Verification items for the finished model (mm, model axes). Face numbers are marked on the shaded views. Coordinates: 2 decimals unless noted, no trailing zeros. Order: outer loops, then holes, each group sorted by start corner. A loop starts at its lowest first (then second) coordinate and runs counter-clockwise, first axis right, second up. Notation, with made-up numbers: M 28,-22.5 L 72,-22.5 A32 cw 72,7.5 Z; hole C 17,11 d7. An arc over 180 degrees is marked long. Return JSON: item names as keys, results as strings.
```python
from build123d import *

# Parameters (mm, degrees)
BOX002_W          = 3
BOX002_H          = 176
BOX002_DEPTH      = 26
FILLET001_R       = 2
CYLINDER020_R     = 30
CYLINDER020_DEPTH = 10
CYLINDER019_R     = 30
CYLINDER019_DEPTH = 10
CYLINDER018_R     = 30
CYLINDER018_DEPTH = 10
CYLINDER016_R     = 30
CYLINDER016_DEPTH = 10
CYLINDER017_R     = 70
CYLINDER017_DEPTH = 10
CYLINDER015_R     = 70
CYLINDER015_DEPTH = 10
CYLINDER014_R     = 70
CYLINDER014_DEPTH = 10
CYLINDER013_R     = 70
CYLINDER013_DEPTH = 10
BOX004_W          = 10
BOX004_H          = 24
BOX004_DEPTH      = 15
CYLINDER012_R     = 30
CYLINDER012_DEPTH = 10
CYLINDER011_R     = 30
CYLINDER011_DEPTH = 10
CYLINDER010_R     = 30
CYLINDER010_DEPTH = 10
CYLINDER008_R     = 30
CYLINDER008_DEPTH = 10
CYLINDER009_R     = 70
CYLINDER009_DEPTH = 10
CYLINDER006_R     = 70
CYLINDER006_DEPTH = 10
CYLINDER005_R     = 70
CYLINDER005_DEPTH = 10
CYLINDER004_R     = 70
CYLINDER004_DEPTH = 10
BOX003_W          = 10
BOX003_H          = 24
BOX003_DEPTH      = 15
BOX_W             = 2
BOX_H             = 176
BOX_DEPTH         = 26
CYLINDER_R        = 2
CYLINDER_DEPTH    = 26
CYLINDER001_R     = 2
CYLINDER001_DEPTH = 26
CYLINDER002_R     = 2
CYLINDER002_DEPTH = 176
CYLINDER003_R     = 2
CYLINDER003_DEPTH = 176
BOX001_W          = 3
BOX001_H          = 180
BOX001_DEPTH      = 30
FILLET_R          = 2


with BuildPart() as fillet001:
    # Box002 → Box002 (new body)
    with BuildSketch(Plane(origin=(7, 2, 2), x_dir=(1, 0, 0), z_dir=(0, 0, 1))):
        with Locations((1.5, 88)):
            Rectangle(BOX002_W, BOX002_H)
    extrude(amount=BOX002_DEPTH)

    # Fillet001
    fillet001_edges = [fillet001.edges().sort_by_distance(p)[0] for p in [
        (8.5, 2, 2),
        (8.5, 2, 28),
        (8.5, 178, 2),
        (8.5, 178, 28),
    ]]
    fillet(fillet001_edges, radius=FILLET001_R)


with BuildPart() as fillet001_1:
    # Fillet001 placement: moved
    add(fillet001.part.moved(Location((-5, 0, 0))))


with BuildPart() as cylinder020:
    # Cylinder020 → Cylinder020 (new body)
    with BuildSketch(Plane(origin=(22, -27, 39.5), x_dir=(0, 0, -1), z_dir=(1, 0, 0))):
        Circle(CYLINDER020_R)
    extrude(amount=CYLINDER020_DEPTH)


with BuildPart() as cylinder019:
    # Cylinder019 → Cylinder019 (new body)
    with BuildSketch(Plane(origin=(22, -27, -24.5), x_dir=(0, 0, -1), z_dir=(1, 0, 0))):
        Circle(CYLINDER019_R)
    extrude(amount=CYLINDER019_DEPTH)


with BuildPart() as cylinder018:
    # Cylinder018 → Cylinder018 (new body)
    with BuildSketch(Plane(origin=(22, 27, -24.5), x_dir=(0, 0, -1), z_dir=(1, 0, 0))):
        Circle(CYLINDER018_R)
    extrude(amount=CYLINDER018_DEPTH)


with BuildPart() as cylinder016:
    # Cylinder016 → Cylinder016 (new body)
    with BuildSketch(Plane(origin=(22, 27, 39.5), x_dir=(0, 0, -1), z_dir=(1, 0, 0))):
        Circle(CYLINDER016_R)
    extrude(amount=CYLINDER016_DEPTH)


with BuildPart() as cylinder017:
    # Cylinder017 → Cylinder017 (new body)
    with BuildSketch(Plane(origin=(22, -58, 7.5), x_dir=(0, 0, -1), z_dir=(1, 0, 0))):
        Circle(CYLINDER017_R)
    extrude(amount=CYLINDER017_DEPTH)


with BuildPart() as cylinder015:
    # Cylinder015 → Cylinder015 (new body)
    with BuildSketch(Plane(origin=(22, 58, 7.5), x_dir=(0, 0, -1), z_dir=(1, 0, 0))):
        Circle(CYLINDER015_R)
    extrude(amount=CYLINDER015_DEPTH)


with BuildPart() as cylinder014:
    # Cylinder014 → Cylinder014 (new body)
    with BuildSketch(Plane(origin=(22, 0, 84.5), x_dir=(0, 0, -1), z_dir=(1, 0, 0))):
        Circle(CYLINDER014_R)
    extrude(amount=CYLINDER014_DEPTH)


with BuildPart() as cylinder013:
    # Cylinder013 → Cylinder013 (new body)
    with BuildSketch(Plane(origin=(22, 0, -69.5), x_dir=(0, 0, -1), z_dir=(1, 0, 0))):
        Circle(CYLINDER013_R)
    extrude(amount=CYLINDER013_DEPTH)


with BuildPart() as cut011:
    # Box004 → Box004 (new body)
    with BuildSketch(Plane(origin=(22, -12, 0), x_dir=(1, 0, 0), z_dir=(0, 0, 1))):
        with Locations((5, 12)):
            Rectangle(BOX004_W, BOX004_H)
    extrude(amount=BOX004_DEPTH)

    # Cut006: cut Cylinder013
    add(cylinder013.part, mode=Mode.SUBTRACT)

    # Cut007: cut Cylinder014
    add(cylinder014.part, mode=Mode.SUBTRACT)

    # Common002: intersect Cylinder015
    add(cylinder015.part, mode=Mode.INTERSECT)

    # Common003: intersect Cylinder017
    add(cylinder017.part, mode=Mode.INTERSECT)

    # Cut008: cut Cylinder016
    add(cylinder016.part, mode=Mode.SUBTRACT)

    # Cut009: cut Cylinder018
    add(cylinder018.part, mode=Mode.SUBTRACT)

    # Cut010: cut Cylinder019
    add(cylinder019.part, mode=Mode.SUBTRACT)

    # Cut011: cut Cylinder020
    add(cylinder020.part, mode=Mode.SUBTRACT)


with BuildPart() as cut011_1:
    # Cut011 placement: moved
    add(cut011.part.moved(Location((-25, 22.5, 7.5))))


with BuildPart() as cylinder012:
    # Cylinder012 → Cylinder012 (new body)
    with BuildSketch(Plane(origin=(22, -27, 39.5), x_dir=(0, 0, -1), z_dir=(1, 0, 0))):
        Circle(CYLINDER012_R)
    extrude(amount=CYLINDER012_DEPTH)


with BuildPart() as cylinder011:
    # Cylinder011 → Cylinder011 (new body)
    with BuildSketch(Plane(origin=(22, -27, -24.5), x_dir=(0, 0, -1), z_dir=(1, 0, 0))):
        Circle(CYLINDER011_R)
    extrude(amount=CYLINDER011_DEPTH)


with BuildPart() as cylinder010:
    # Cylinder010 → Cylinder010 (new body)
    with BuildSketch(Plane(origin=(22, 27, -24.5), x_dir=(0, 0, -1), z_dir=(1, 0, 0))):
        Circle(CYLINDER010_R)
    extrude(amount=CYLINDER010_DEPTH)


with BuildPart() as cylinder008:
    # Cylinder008 → Cylinder008 (new body)
    with BuildSketch(Plane(origin=(22, 27, 39.5), x_dir=(0, 0, -1), z_dir=(1, 0, 0))):
        Circle(CYLINDER008_R)
    extrude(amount=CYLINDER008_DEPTH)


with BuildPart() as cylinder009:
    # Cylinder009 → Cylinder009 (new body)
    with BuildSketch(Plane(origin=(22, -58, 7.5), x_dir=(0, 0, -1), z_dir=(1, 0, 0))):
        Circle(CYLINDER009_R)
    extrude(amount=CYLINDER009_DEPTH)


with BuildPart() as cylinder006:
    # Cylinder006 → Cylinder006 (new body)
    with BuildSketch(Plane(origin=(22, 58, 7.5), x_dir=(0, 0, -1), z_dir=(1, 0, 0))):
        Circle(CYLINDER006_R)
    extrude(amount=CYLINDER006_DEPTH)


with BuildPart() as cylinder005:
    # Cylinder005 → Cylinder005 (new body)
    with BuildSketch(Plane(origin=(22, 0, 84.5), x_dir=(0, 0, -1), z_dir=(1, 0, 0))):
        Circle(CYLINDER005_R)
    extrude(amount=CYLINDER005_DEPTH)


with BuildPart() as cylinder:
    # Cylinder004 → Cylinder004 (new body)
    with BuildSketch(Plane(origin=(22, 0, -69.5), x_dir=(0, 0, -1), z_dir=(1, 0, 0))):
        Circle(CYLINDER004_R)
    extrude(amount=CYLINDER004_DEPTH)


with BuildPart() as cut005:
    # Box003 → Box003 (new body)
    with BuildSketch(Plane(origin=(22, -12, 0), x_dir=(1, 0, 0), z_dir=(0, 0, 1))):
        with Locations((5, 12)):
            Rectangle(BOX003_W, BOX003_H)
    extrude(amount=BOX003_DEPTH)

    # Cut: cut Cylinder
    add(cylinder.part, mode=Mode.SUBTRACT)

    # Cut001: cut Cylinder005
    add(cylinder005.part, mode=Mode.SUBTRACT)

    # Common: intersect Cylinder006
    add(cylinder006.part, mode=Mode.INTERSECT)

    # Common001: intersect Cylinder009
    add(cylinder009.part, mode=Mode.INTERSECT)

    # Cut002: cut Cylinder008
    add(cylinder008.part, mode=Mode.SUBTRACT)

    # Cut003: cut Cylinder010
    add(cylinder010.part, mode=Mode.SUBTRACT)

    # Cut004: cut Cylinder011
    add(cylinder011.part, mode=Mode.SUBTRACT)

    # Cut005: cut Cylinder012
    add(cylinder012.part, mode=Mode.SUBTRACT)


with BuildPart() as cut005_1:
    # Cut005 placement: moved
    add(cut005.part.moved(Location((-25, 157.5, 7.5))))


with BuildPart() as cube001:
    # Box → Box (new body)
    with BuildSketch(Plane(origin=(0, 2, 2), x_dir=(1, 0, 0), z_dir=(0, 0, 1))):
        with Locations((1, 88)):
            Rectangle(BOX_W, BOX_H)
    extrude(amount=BOX_DEPTH)


with BuildPart() as cylinder001:
    # Cylinder → Cylinder (new body)
    with BuildSketch(Plane(origin=(2, 2, 2), x_dir=(0, 1, 0), z_dir=(0, 0, 1))):
        Circle(CYLINDER_R)
    extrude(amount=CYLINDER_DEPTH)


with BuildPart() as cylinder002:
    # Cylinder001 → Cylinder001 (new body)
    with BuildSketch(Plane(origin=(2, 178, 2), x_dir=(0, 1, 0), z_dir=(0, 0, 1))):
        Circle(CYLINDER001_R)
    extrude(amount=CYLINDER001_DEPTH)


with BuildPart() as cylinder003:
    # Cylinder002 → Cylinder002 (new body)
    with BuildSketch(Plane(origin=(2, 178, 2), x_dir=(1, 0, 0), z_dir=(0, -1, 0))):
        Circle(CYLINDER002_R)
    extrude(amount=CYLINDER002_DEPTH)


with BuildPart() as cylinder004:
    # Cylinder003 → Cylinder003 (new body)
    with BuildSketch(Plane(origin=(2, 178, 28), x_dir=(1, 0, 0), z_dir=(0, -1, 0))):
        Circle(CYLINDER003_R)
    extrude(amount=CYLINDER003_DEPTH)


with BuildPart() as sphere001:
    # Sphere → Sphere (revolve)
    with BuildSketch(Plane(origin=(2, 2, 2), x_dir=(1, 0, 0), z_dir=(0, -1, 0))):
        with BuildLine():
            ThreePointArc((0, -2), (2, 0), (0, 2))
            Line((0, 2), (0, -2))
        make_face()
    revolve(axis=Axis((2, 2, 2), (0, 0, 1)))


with BuildPart() as sphere002:
    # Sphere001 → Sphere001 (revolve)
    with BuildSketch(Plane(origin=(2, 178, 2), x_dir=(1, 0, 0), z_dir=(0, -1, 0))):
        with BuildLine():
            ThreePointArc((0, -2), (2, 0), (0, 2))
            Line((0, 2), (0, -2))
        make_face()
    revolve(axis=Axis((2, 178, 2), (0, 0, 1)))


with BuildPart() as sphere003:
    # Sphere002 → Sphere002 (revolve)
    with BuildSketch(Plane(origin=(2, 2, 28), x_dir=(1, 0, 0), z_dir=(0, -1, 0))):
        with BuildLine():
            ThreePointArc((0, -2), (2, 0), (0, 2))
            Line((0, 2), (0, -2))
        make_face()
    revolve(axis=Axis((2, 2, 28), (0, 0, 1)))


with BuildPart() as sphere004:
    # Sphere003 → Sphere003 (revolve)
    with BuildSketch(Plane(origin=(2, 178, 28), x_dir=(1, 0, 0), z_dir=(0, -1, 0))):
        with BuildLine():
            ThreePointArc((0, -2), (2, 0), (0, 2))
            Line((0, 2), (0, -2))
        make_face()
    revolve(axis=Axis((2, 178, 28), (0, 0, 1)))


with BuildPart() as cut014:
    # Box001 → Box001 (new body)
    with BuildSketch(Plane(origin=(2, 0, 0), x_dir=(1, 0, 0), z_dir=(0, 0, 1))):
        with Locations((1.5, 90)):
            Rectangle(BOX001_W, BOX001_H)
    extrude(amount=BOX001_DEPTH)

    # Fillet
    fillet_edges = [cut014.edges().sort_by_distance(p)[0] for p in [
        (3.5, 0, 0),
        (3.5, 0, 30),
        (3.5, 180, 0),
        (3.5, 180, 30),
    ]]
    fillet(fillet_edges, radius=FILLET_R)

    # Fusion: union Cube001, Cylinder001, Cylinder002, Cylinder003, Cylinder004, Sphere001, Sphere002, Sphere003, Sphere004
    add(cube001.part)
    add(cylinder001.part)
    add(cylinder002.part)
    add(cylinder003.part)
    add(cylinder004.part)
    add(sphere001.part)
    add(sphere002.part)
    add(sphere003.part)
    add(sphere004.part)

    # Cut012: cut Cut005
    add(cut005_1.part, mode=Mode.SUBTRACT)

    # Cut013: cut Cut011
    add(cut011_1.part, mode=Mode.SUBTRACT)

    # Cut014: cut Fillet001
    add(fillet001_1.part, mode=Mode.SUBTRACT)


solid = cut014.part
```
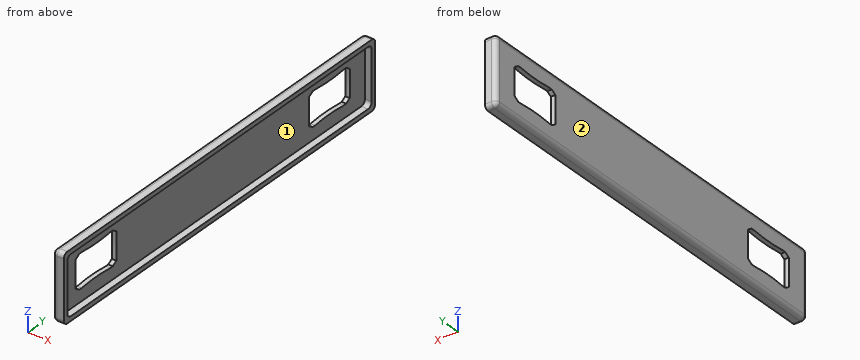
Q1. Draft check along Y on the marked faces 1 and 2. Enter one of: pulls with the +Y half, pulls with the -Y half, needs draft (parallel to the pull), parting line crosses it, or undercut.
Values:
{"face 1": "undercut", "face 2": "needs draft"}
Q2. Material ranges on line 1 along Z through (x, y) = (4.6, 115); line 2 along Y through (x, z) = (3.4, 11.5); line 3 along Y through (x, z) = (0.65, 21.25), recorded low to high.
Values:
{"line 1": "0 to 2, 28 to 30", "line 2": "0 to 2, 178 to 180", "line 3": "0.52 to 10.89, 34.11 to 145.89, 169.11 to 179.48"}
Q3. Go/stop test with flat-tipped pins: pin 1 (1.1 mm diameter, centred on x = 1, y = 31.5, fed in from +Z); pin 2 (1.1 mm diameter, centred on x = 0.5, y = 166.5, fed in from -Z); pin 3 (10 mm diameter, centred on y = 152.5, z = 20.5, fed in from +X). Record where each tip stops, or that it passes through.
Values:
{"pin 1": "z = 29.95", "pin 2": "z = 0.24", "pin 3": "x = 2"}
Q4. Cross-section at D-D, the plane z = 12. Record the boundary of the cut face in (x, y).
Values:
{"outline": "M 0,2 A2 ccw 2,0 L 5,0 L 5,2 L 2,2 L 2,10.56 L 0,10.56 Z; M 0,34.44 L 2,34.44 L 2,145.56 L 0,145.56 Z; M 0,169.44 L 2,169.44 L 2,178 L 5,178 L 5,180 L 2,180 A2 ccw 0,178 Z"}
Q5. Cross-section at A-A, the plane x = 3.7. Record the boundary of the cut face in (y, z).
Values:
{"outline": "M 0,2 A2 ccw 2,0 L 178,0 A2 ccw 180,2 L 180,28 A2 ccw 178,30 L 2,30 A2 ccw 0,28 Z; hole M 2,4 A2 ccw 4,2 L 176,2 A2 ccw 178,4 L 178,26 A2 ccw 176,28 L 4,28 A2 ccw 2,26 Z"}
Q6. Cross-section at C-C, the plane z = 5.5. Record the boundary of the cut face in (x, y).
Values:
{"outline": "M 0,2 A2 ccw 2,0 L 5,0 L 5,2 L 2,2 L 2,178 L 5,178 L 5,180 L 2,180 A2 ccw 0,178 Z"}
Q7. Cross-section at B-B, the plane y = 19. Record the boundary of the cut face in (x, z).
Values:
{"outline": "M 0,2 A2 ccw 2,0 L 5,0 L 5,2 L 2,2 L 2,7.91 L 0,7.91 Z; M 0,22.09 L 2,22.09 L 2,28 L 5,28 L 5,30 L 2,30 A2 ccw 0,28 Z"}
